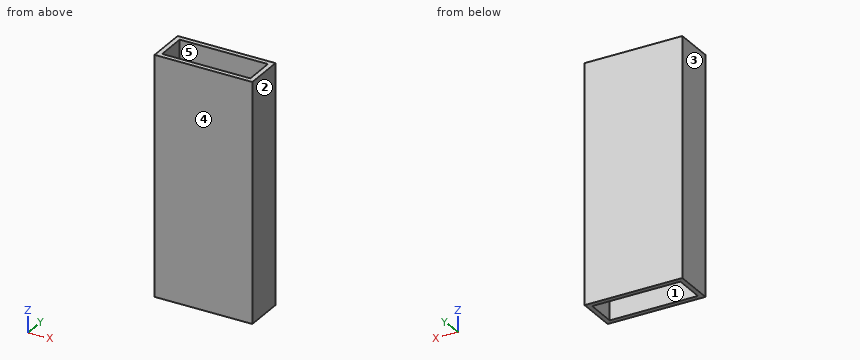
Autodesk Inventor part; units mm, degrees
ref_plane "YZ Plane" through (0, 0, 0) normal (1, 0, 0) x (0, 1, 0)
ref_plane "XZ Plane" through (0, 0, 0) normal (0, 1, 0) x (-1, 0, 0)
ref_plane "XY Plane" through (0, 0, 0) normal (0, 0, 1) x (1, 0, 0)
sketch "Boceto1" plane through (0, 0, 0) normal (0, 1, 0) x (-1, 0, 0)
  line L0 (15.5342, 31.1771) -> (-21.4658, 31.1771)
  line L1 (-21.4658, 31.1771) -> (-21.4658, -58.8229)
  line L2 (-21.4658, -58.8229) -> (15.5342, -58.8229)
  line L3 (15.5342, -58.8229) -> (15.5342, 31.1771)
  point P0 (0, 0)
  dimension "d0" = 37
  dimension "d1" = 90
extrude "Extrusión1" add sketch "Boceto1" along normal blind 15
sketch "Boceto2" plane through (-15.5342, 0, 31.1771) normal (0, 0, 1) x (1, 0, 0)
  line L0 (1.8, 13.2) -> (35.2, 13.2)
  line L1 (35.2, 13.2) -> (35.2, 1.8)
  line L2 (35.2, 1.8) -> (1.8, 1.8)
  line L3 (1.8, 1.8) -> (1.8, 13.2)
  line L4 (0, 15) -> (37, 15)
  line L5 (0, 0) -> (37, 0)
  line L6 (0, 0) -> (0, 15)
  line L7 (37, 0) -> (37, 15)
  point P0 (15.5342, 0)
  dimension "d4" = 1.8
  dimension "d5" = 1.8
  dimension "d6" = 1.8
  dimension "d7" = 1.8
  dimension "d8" = 33.4
  dimension "d9" = 11.4
extrude "Extrusión2" cut sketch "Boceto2" against normal blind 90 contours L0 L1 L2 L3
properties part number "caja_grafeno"
The model under review builds one solid part; all positions refer to its coordinate system, in mm. Face numbers are marked on the shaded views. A direction names the side the tool comes from. Round coordinates to 2 decimals unless told otherwise and drop trailing zeros. Order: outer loops, then holes, each group sorted by start corner. A loop starts at its lowest first (then second) coordinate and runs counter-clockwise, first axis right, second up. Notation, with made-up numbers: (-21, -19) -> (-5, -19) arc R27 ccw to (-5, 20) -> close; hole circle Ø11 at (-35, 89). An arc over 180 degrees is marked (long way). Write item = value, one per line. Start each with the question number.
Item 1: Consider section B-B on y = 8.5. Write out the cut boundary in (x, z).
Item 2: Consider section A-A on x = -11. Write out the cut boundary in (y, z).
Item 3: For the marked faces 4 and 5, list the 3-axis set-ups (+Z, -Z, +X, -X, +Y, -Y) from which the entire face can be reached by the end or side of a thin tool; tool diameter is ignored.
Item 4: For line 1 along Y through (x, z) = (8, 25); line 2 along X through (y, z) = (12.5, -12), list the stretches that pass through material, from the lowest coordinate up.
Item 5: Mouldability with a two-part tool opening along X and no side actions: class the marked faces 1, 2 and 3 as released by +X, released by -X, zero draft, split by the parting line, or undercut.
Item 6: Consider section C-C on z = -41.5. Write out the cut boundary in (x, y), plus the area to 3 significant figures.
Item 7: Clearance check with a flat-ended pin moving along its axis: pin 1 Ø3 at (x, y) = (1.5, 13) entering from -Z. State where the tip first meets the part, or that it passes through.
Conclusion:
q1.outline = (-15.53, -58.82) -> (-13.73, -58.82) -> (-13.73, 31.18) -> (-15.53, 31.18) -> close; (19.67, -58.82) -> (21.47, -58.82) -> (21.47, 31.18) -> (19.67, 31.18) -> close
q2.outline = (0, -58.82) -> (1.8, -58.82) -> (1.8, 31.18) -> (0, 31.18) -> close; (13.2, -58.82) -> (15, -58.82) -> (15, 31.18) -> (13.2, 31.18) -> close
q3.face_4 = +Z, -Z, +X, -X, -Y
q3.face_5 = +Z, -Z
q4.line_1 = 0 to 1.8, 13.2 to 15
q4.line_2 = -15.53 to -13.73, 19.67 to 21.47
q5.face_1 = undercut
q5.face_2 = released by +X
q5.face_3 = released by -X
q6.outline = (-15.53, 0) -> (21.47, 0) -> (21.47, 15) -> (-15.53, 15) -> close; hole (-13.73, 1.8) -> (19.67, 1.8) -> (19.67, 13.2) -> (-13.73, 13.2) -> close
q6.area = 174 mm2
q7.pin_1 = -58.82
